Verification items for the finished model (mm, model axes). A direction names the side the tool comes from. Round coordinates to 2 decimals unless told otherwise and drop trailing zeros. Write each loop counter-clockwise with the first axis right and the second up, starting at its lowest first coordinate (ties: lowest second). Pieces come first, ordered by that corner, then holes. Notation, with made-up numbers: M 86,6 L 96,6 A35 ccw 96,38 Z; hole C 60.5,55 d1. An arc over 180 degrees is marked long. Write each question's results on one line, items separated by ' | '.
from build123d import *

# Parameters (mm, degrees)
SKETCH1_W           = 120
SKETCH1_H           = 30
BOSS_EXTRUDE1_DEPTH = 80
SHELL1_T            = -5
SKETCH2_R           = 4.17592015
CUT_EXTRUDE1_DEPTH  = 15
LPATTERN1_COUNT     = 4
LPATTERN1_PITCH     = 110


with BuildPart() as part:
    # Sketch1 → Boss-Extrude1 (new body)
    with BuildSketch(Plane.XY):
        with Locations((14.869684499, 8.141289438)):
            Rectangle(SKETCH1_W, SKETCH1_H)
    extrude(amount=BOSS_EXTRUDE1_DEPTH)

    # Shell1
    shell1_openings = [part.faces().sort_by_distance(p)[0] for p in [
        (14.869684499, -6.858710562, 40),
    ]]
    offset(amount=SHELL1_T, openings=shell1_openings, kind=Kind.INTERSECTION)

    # Sketch2 → Cut-Extrude1 (cut)
    with BuildSketch(Plane(origin=(0, 0, 0), x_dir=(-1, 0, 0), z_dir=(0, 0, -1))):
        with Locations((30.130315501, 7.814471991)):
            Circle(SKETCH2_R)
    cut_extrude1 = extrude(amount=-CUT_EXTRUDE1_DEPTH, mode=Mode.SUBTRACT)

    # LPattern1: Cut-Extrude1 ×4
    with Locations(*[(-i * LPATTERN1_PITCH, 0, 0) for i in range(1, LPATTERN1_COUNT)]):
        add(cut_extrude1, mode=Mode.SUBTRACT)


solid = part.part
1) Access from +Z, -Z, +X, -X, +Y, -Y to the whole of each face (thin tool, end or side, straight path). Record for faces 4 (the flat face through (14, 6, 75)), 5 (the cylindrical face through (-29.587, 11.955, 2.465)), 6 (the flat face through (10.1, -6.859, 75.4)).
Calculated:
face 4: -Y | face 5: -Z | face 6: +Z, -Z, +X, -X, -Y
2) Material ranges on line 1 (Z direction, x = -2.5, y = 3.75); line 2 (X direction, y = 4.5, z = 15.5); line 3 (Y direction, x = -29, z = 69.5), recorded low to high. Write a range as [from, to].
Calculated:
line 1: z = [0, 5], [75, 80] | line 2: x = [-45.13, -40.13], [69.87, 74.87] | line 3: y = [18.14, 23.14]
3) Sectioned sample at D-D, the plane x = -28. Record the cut outline in (y, z).
Calculated:
outline: M -6.86,0 L 4.22,0 L 4.22,5 L -6.86,5 Z; M -6.86,75 L 18.14,75 L 18.14,5 L 11.41,5 L 11.41,0 L 23.14,0 L 23.14,80 L -6.86,80 Z
4) Depth check by flat-ended pin: P1, Ø2, axis at x = 61, z = 54, coming from the -Y side. Enter the tip coordinate at first touch or a pass-through.
Calculated:
P1: stops at y = 18.14
5) Sectioned sample at A-A, the plane y = 16. Record the cut outline in (x, z).
Calculated:
outline: M -45.13,0 L 74.87,0 L 74.87,80 L -45.13,80 Z; hole M -40.13,5 L 69.87,5 L 69.87,75 L -40.13,75 Z
6) Sectioned sample at C-C, the plane z = 73. Record the cut outline in (x, y), and give its area (3 significant figures).
Calculated:
outline: M -45.13,-6.86 L -40.13,-6.86 L -40.13,18.14 L 69.87,18.14 L 69.87,-6.86 L 74.87,-6.86 L 74.87,23.14 L -45.13,23.14 Z | area: 850 mm²
7) Sectioned sample at B-B, the plane x = 67. Record the cut outline in (y, z), and give its area (3 significant figures).
Calculated:
outline: M -6.86,0 L 23.14,0 L 23.14,80 L -6.86,80 L -6.86,75 L 18.14,75 L 18.14,5 L -6.86,5 Z | area: 650 mm²
8) Draft check along X on faces 1 (the flat face through (69.87, 5, 40)), 2 (the flat face through (14, 23.141, 39)), 3 (the flat face through (-45.13, 8, 39)). Enter one of: pulls with the +X half, pulls with the -X half, needs draft (parallel to the pull), parting line crosses it, or undercut.
Calculated:
face 1: undercut | face 2: needs draft | face 3: pulls with the -X half
